Here's how the part is built. I have some questions about the finished solid (model axes, mm). Round coordinates to 2 decimals unless told otherwise and drop trailing zeros. Order: outer loops, then holes, each group sorted by start corner. A loop starts at its lowest first (then second) coordinate and runs counter-clockwise, first axis right, second up. Notation, with made-up numbers: (72, 76) -> (106, 76) arc R18 cw to (106, 111) -> close; hole circle Ø11 at (-3.5, 54.25). An arc over 180 degrees is marked (long way). Use a Markdown table: item, result. Add a question column.
(1) If I drill on probe 1 along X at (y, z) = (-134.5, 0.7); probe 2 along Y at (x, z) = (-90, 1.95); probe 3 along Y at (x, z) = (-129.5, 1.35), over which ranges is the centre line in solid material (lowest first)?
(2) I'm going to push a flat-ended pin straight in: P1, Ø1.5, axis at y = 91.5, z = 3.5, coming from the +X side. Where does the tip first touch, or does it pass through?
(3) I want a section at A-A, the plane y = 17. Please give me the cut outline in (x, z).
(4) I want a section at B-B, the plane z = 1.05. Give the number of separate pieces and of enclosed holes in the cut face, then the cut area to 3 significant figures.
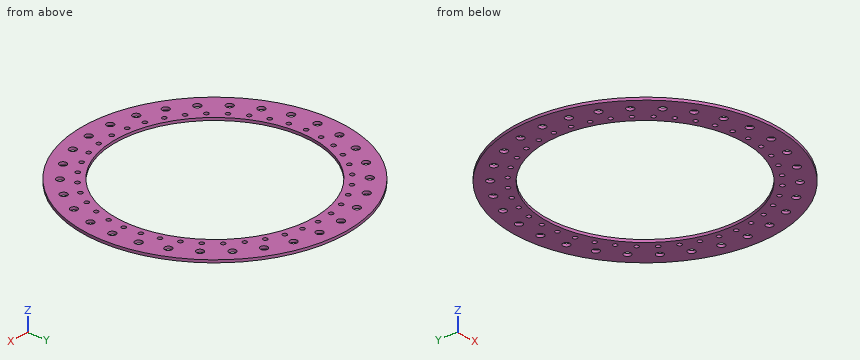
from build123d import *

# Parameters (mm, degrees)
CROQUIS1_R                   = 200
CROQUIS1_R_2                 = 150
CROQUIS1_R_3                 = 5.4
SALIENTE_EXTRUIR1_DEPTH      = 4
TALADRO_DE_MARGEN_PARA_M61_D = 6.6


with BuildPart() as part:
    # Croquis1 → Saliente-Extruir1 (new body)
    with BuildSketch(Plane.XY):
        Circle(CROQUIS1_R)
        Circle(CROQUIS1_R_2, mode=Mode.SUBTRACT)
        with Locations((145.623058987, 105.801345413)):
            Circle(CROQUIS1_R_3, mode=Mode.SUBTRACT)
        with Locations((164.438182376, 73.212595754)):
            Circle(CROQUIS1_R_3, mode=Mode.SUBTRACT)
        with Locations((176.066568132, 37.424104347)):
            Circle(CROQUIS1_R_3, mode=Mode.SUBTRACT)
        with Locations((180, 0)):
            Circle(CROQUIS1_R_3, mode=Mode.SUBTRACT)
        with Locations((176.066568132, -37.424104347)):
            Circle(CROQUIS1_R_3, mode=Mode.SUBTRACT)
        with Locations((164.438182376, -73.212595754)):
            Circle(CROQUIS1_R_3, mode=Mode.SUBTRACT)
        with Locations((145.623058987, -105.801345413)):
            Circle(CROQUIS1_R_3, mode=Mode.SUBTRACT)
        with Locations((120.443509145, -133.766068586)):
            Circle(CROQUIS1_R_3, mode=Mode.SUBTRACT)
        with Locations((90, -155.884572681)):
            Circle(CROQUIS1_R_3, mode=Mode.SUBTRACT)
        with Locations((55.623058987, -171.190172933)):
            Circle(CROQUIS1_R_3, mode=Mode.SUBTRACT)
        with Locations((18.815123388, -179.013941166)):
            Circle(CROQUIS1_R_3, mode=Mode.SUBTRACT)
        with Locations((-18.815123388, -179.013941166)):
            Circle(CROQUIS1_R_3, mode=Mode.SUBTRACT)
        with Locations((-55.623058987, -171.190172933)):
            Circle(CROQUIS1_R_3, mode=Mode.SUBTRACT)
        with Locations((-90, -155.884572681)):
            Circle(CROQUIS1_R_3, mode=Mode.SUBTRACT)
        with Locations((-120.443509145, -133.766068586)):
            Circle(CROQUIS1_R_3, mode=Mode.SUBTRACT)
        with Locations((-145.623058987, -105.801345413)):
            Circle(CROQUIS1_R_3, mode=Mode.SUBTRACT)
        with Locations((-164.438182376, -73.212595754)):
            Circle(CROQUIS1_R_3, mode=Mode.SUBTRACT)
        with Locations((-176.066568132, -37.424104347)):
            Circle(CROQUIS1_R_3, mode=Mode.SUBTRACT)
        with Locations((-180, 0)):
            Circle(CROQUIS1_R_3, mode=Mode.SUBTRACT)
        with Locations((-176.066568132, 37.424104347)):
            Circle(CROQUIS1_R_3, mode=Mode.SUBTRACT)
        with Locations((-164.438182376, 73.212595754)):
            Circle(CROQUIS1_R_3, mode=Mode.SUBTRACT)
        with Locations((-145.623058987, 105.801345413)):
            Circle(CROQUIS1_R_3, mode=Mode.SUBTRACT)
        with Locations((-120.443509145, 133.766068586)):
            Circle(CROQUIS1_R_3, mode=Mode.SUBTRACT)
        with Locations((-90, 155.884572681)):
            Circle(CROQUIS1_R_3, mode=Mode.SUBTRACT)
        with Locations((-55.623058987, 171.190172933)):
            Circle(CROQUIS1_R_3, mode=Mode.SUBTRACT)
        with Locations((-18.815123388, 179.013941166)):
            Circle(CROQUIS1_R_3, mode=Mode.SUBTRACT)
        with Locations((18.815123388, 179.013941166)):
            Circle(CROQUIS1_R_3, mode=Mode.SUBTRACT)
        with Locations((55.623058987, 171.190172933)):
            Circle(CROQUIS1_R_3, mode=Mode.SUBTRACT)
        with Locations((90, 155.884572681)):
            Circle(CROQUIS1_R_3, mode=Mode.SUBTRACT)
        with Locations((120.443509145, 133.766068586)):
            Circle(CROQUIS1_R_3, mode=Mode.SUBTRACT)
    extrude(amount=SALIENTE_EXTRUIR1_DEPTH)

    # Taladro de margen para M61 (through all)
    with Locations(Plane(origin=(-113.13708499, 113.13708499, 0), x_dir=(-1, 0, 0), z_dir=(0, 0, -1))):
        with Locations((0, 0), (-19.091444623, 16.30563411), (-40.498605032, 29.42395888), (-63.69436589, 39.031957617), (16.30563411, -19.091444623), (29.42395888, -40.498605032), (39.031957617, -63.69436589), (44.893049505, -88.107570584), (46.86291501, -113.13708499), (44.893049505, -138.166599396), (39.031957617, -162.57980409), (29.42395888, -185.775564948), (16.30563411, -207.182725357), (0, -226.27416998), (-19.091444623, -242.57980409), (-40.498605032, -255.69812886), (-63.69436589, -265.306127597), (-88.107570584, -271.167219485), (-113.13708499, -273.13708499), (-138.166599396, -271.167219485), (-162.57980409, -265.306127597), (-185.775564948, -255.69812886), (-207.182725357, -242.57980409), (-226.27416998, -226.27416998), (-242.57980409, -207.182725357), (-255.69812886, -185.775564948), (-265.306127597, -162.57980409), (-271.167219485, -138.166599396), (-273.13708499, -113.13708499), (-271.167219485, -88.107570584), (-265.306127597, -63.69436589), (-255.69812886, -40.498605032), (-242.57980409, -19.091444623), (-226.27416998, 0), (-207.182725357, 16.30563411), (-185.775564948, 29.42395888), (-162.57980409, 39.031957617), (-138.166599396, 44.893049505), (-113.13708499, 46.86291501), (-88.107570584, 44.893049505)):
            Hole(TALADRO_DE_MARGEN_PARA_M61_D / 2)


solid = part.part
Taken from the geometry:
| question | item | result |
|---|---|---|
| 1 | probe 1 | x = -148.02 to -125.79, -115.09 to -66.41, 66.41 to 115.09, 125.79 to 148.02 |
| 1 | probe 2 | y = -178.61 to -161.28, -150.48 to -120, 120 to 150.48, 161.28 to 178.61 |
| 1 | probe 3 | y = -152.41 to -97.35, -90.75 to -75.7, 75.7 to 90.75, 97.35 to 152.41 |
| 2 | P1 | stops at x = 178.23 |
| 3 | outline | (-199.28, 0) -> (-149.03, 0) -> (-149.03, 4) -> (-199.28, 4) -> close; (149.03, 0) -> (199.28, 0) -> (199.28, 4) -> (149.03, 4) -> close |
| 4 | separate pieces | 1 |
| 4 | enclosed holes | 71 |
| 4 | area | 50,900 mm2 |
